Geometry: see drawing. Coordinates: mm, zero at the bounding-box minimum. A direction names the side the tool comes from. Round coordinates to 2 decimals unless told otherwise and drop trailing zeros. Write each loop counter-clockwise with the first axis right and the second up, starting at its lowest first coordinate (ties: lowest second). Pieces come first, ordered by that corner, then holes. Notation, with made-up numbers: M -35.5,30 L 11.5,30 A18 ccw 11.5,55 Z; hole C 80,-29.75 d8. An arc over 180 degrees is marked long. Use one line per item in the form item = value. Start each with the question number.
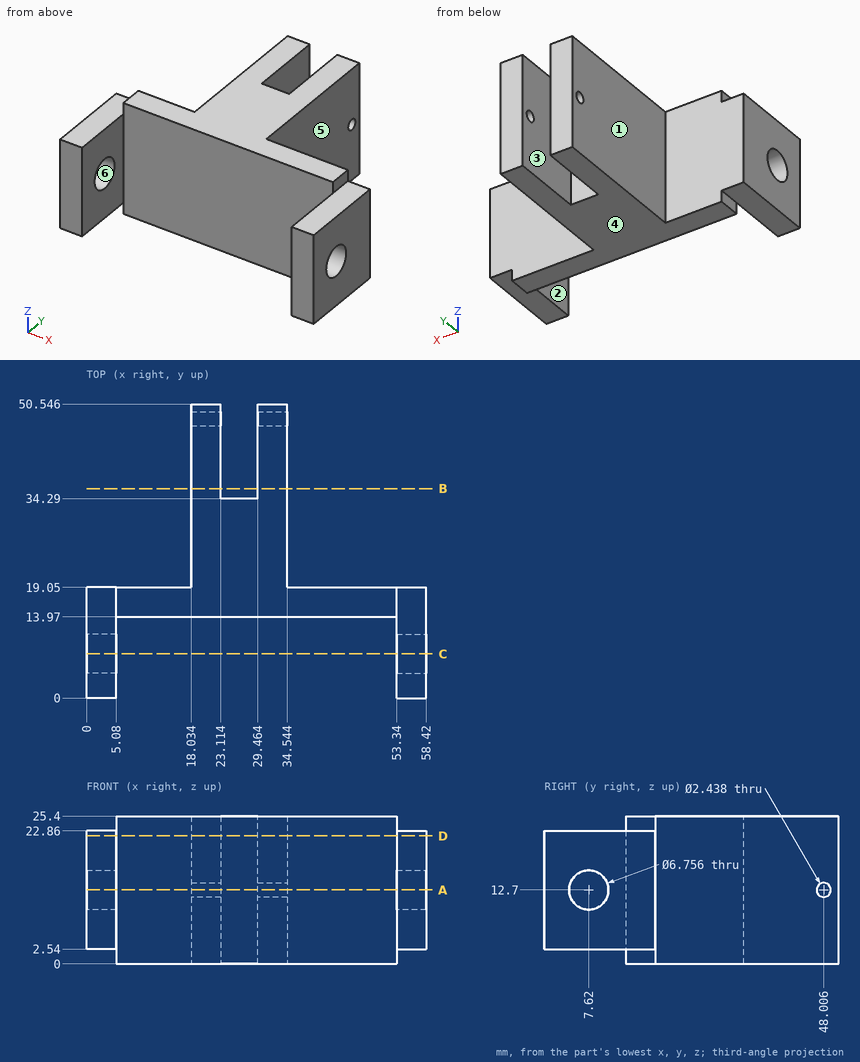
Item 1: Ray query, line 1 (Y direction, x = 3.95, z = 12.7); line 2 (X direction, y = 10, z = 8.5); line 3 (X direction, y = 43.5, z = 21.75). Return the intervals inside material, ascending. Write a range as from..to.
Item 2: Cut plane B-B (y = 36). Output: boundary loops of the cut face in (x, z).
Item 3: Reachability of the marked faces 1, 2 and 3 from +Z, -Z, +X, -X, +Y, -Y: full face, straight path, thin tool, end or side. Return the list, or none.
Item 4: Draft query along Z for the marked faces 4, 5 and 6. Return one class per face: +Z half, -Z half, draft (parallel to the pull), parting line (faces both ways), or undercut.
Item 5: First-contact query: pin 1 (1.5 mm diameter, centred on x = 1.5, y = 11.5, fed in from -Z); pin 2 (6 mm diameter, centred on y = 41.5, z = 18.5, fed in from -X); pin 3 (8 mm diameter, centred on y = 42, z = 14.5, fed in from +X). Flat tips, straight axial feed; report the tip coordinate or a pass-through.
Item 6: Cut plane D-D (z = 22). Output: boundary loops of the cut face in (x, y).
Item 7: Cut plane C-C (y = 7.62). Output: boundary loops of the cut face in (x, z), plus the area to 3 significant figures.
Item 8: Cut plane A-A (z = 12.7). Give the number of separate pieces and of enclosed holes in the cut face, plus the area to 3 significant figures.
Final values:
q1.line_1 = 0..4.24, 11..19.05
q1.line_2 = 0..5.08, 53.34..58.42
q1.line_3 = 18.03..23.11, 29.46..34.54
q2.outline = M 18.03,0 L 23.11,0 L 23.11,25.4 L 18.03,25.4 Z; M 29.46,0 L 34.54,0 L 34.54,25.4 L 29.46,25.4 Z
q3.face_1 = +Z, -Z, -X, +Y
q3.face_2 = +Z, -Z, -Y
q3.face_3 = +Z, -Z, +Y
q4.face_4 = -Z half
q4.face_5 = draft
q4.face_6 = undercut
q5.pin_1 = 2.54
q5.pin_2 = 18.03
q5.pin_3 = 34.54
q6.outline = M 0,0 L 5.08,0 L 5.08,13.97 L 53.34,13.97 L 53.34,0 L 58.42,0 L 58.42,19.05 L 34.54,19.05 L 34.54,50.55 L 29.46,50.55 L 29.46,34.29 L 23.11,34.29 L 23.11,50.55 L 18.03,50.55 L 18.03,19.05 L 0,19.05 Z
q7.outline = M 0,2.54 L 5.08,2.54 L 5.08,9.32 L 0,9.32 Z; M 0,16.08 L 5.08,16.08 L 5.08,22.86 L 0,22.86 Z; M 53.34,2.54 L 58.42,2.54 L 58.42,9.32 L 53.34,9.32 Z; M 53.34,16.08 L 58.42,16.08 L 58.42,22.86 L 53.34,22.86 Z
q7.area = 138 mm^2
q8.separate_pieces = 5
q8.enclosed_holes = 0
q8.area = 762 mm^2
